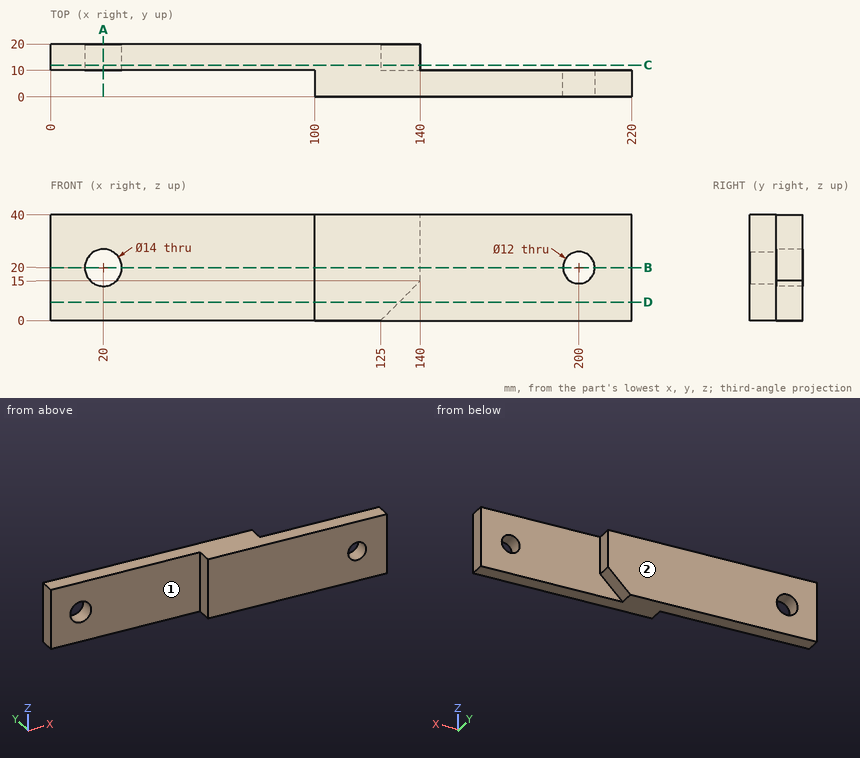
Drawing for the job (mm, zero at the part's lowest x, y, z). A direction names the side the tool comes from. Round coordinates to 2 decimals unless told otherwise and drop trailing zeros. Write each loop counter-clockwise with the first axis right and the second up, starting at its lowest first coordinate (ties: lowest second). Pieces come first, ordered by that corner, then holes.
Item 1: Drop flat-ended pins along their axis: pin 1 Ø4 at (x, z) = (64, 28.5) entering from -Y; pin 2 Ø4 at (y, z) = (17.5, 23) entering from +X; pin 3 Ø20 at (x, z) = (162, 16.5) entering from +Y. Give the stop position or say it passes through.
Filled in:
pin 1: stops at y = 10
pin 2: stops at x = 140
pin 3: stops at y = 10
Item 2: Band-saw the part on D-D on z = 7. Write the cut outline in (x, y).
Filled in:
outline: (0, 10) - (100, 10) - (100, 0) - (220, 0) - (220, 10) - (132, 10) - (132, 20) - (0, 20) - close
Item 3: Band-saw the part on B-B on z = 20. Write the cut outline in (x, y), then the cut area to 3 significant figures.
Filled in:
outline: (0, 10) - (13, 10) - (13, 20) - (0, 20) - close; (27, 10) - (100, 10) - (100, 0) - (194, 0) - (194, 10) - (140, 10) - (140, 20) - (27, 20) - close; (206, 0) - (220, 0) - (220, 10) - (206, 10) - close
area: 2,340 mm2
Item 4: Band-saw the part on A-A on x = 20. Write the cut outline in (y, z), then the cut area to 3 significant figures.
Filled in:
outline: (10, 0) - (20, 0) - (20, 13) - (10, 13) - close; (10, 27) - (20, 27) - (20, 40) - (10, 40) - close
area: 260 mm2
Item 5: Band-saw the part on C-C on y = 12. Write the cut outline in (x, z), then the cut area to 3 significant figures.
Filled in:
outline: (0, 0) - (125, 0) - (140, 15) - (140, 40) - (0, 40) - close; hole circle Ø14 at (20, 20)
area: 5,330 mm2
Item 6: Drill centre lines: L1, parallel to Z at x = 20, y = 17.25; L2, parallel to Z at x = 200, y = 3; L3, parallel to X at y = 1.75, z = 34.5. Where is each one in solid material? Low to high.
Filled in:
L1: z = 0 to 13, 27 to 40
L2: z = 0 to 14, 26 to 40
L3: x = 100 to 220
Item 7: Tool access for the marked faces 1 and 2: list every direction of +Z, -Z, +X, -X, +Y, -Y with a clear straight run to the whole face (end or side of a thin tool).
Filled in:
face 1: +Z, -Z, -X, -Y
face 2: +Z, -Z, +X, -X, +Y
